Geometry: final body of the model. Coordinates: model frame, mm. Round coordinates to 2 decimals unless told otherwise and drop trailing zeros. Loops run counter-clockwise (first coordinate to the right, second up) from the corner with the lowest first, then second, coordinate; pieces in that order, holes last. Notation, with made-up numbers: (-39.75, 15.25) - (18.25, 15.25) arc R10 cw to (18.25, 32.25) - close; hole circle Ø7 at (11.25, 29.25). An arc over 180 degrees is marked (long way). Return JSON: item names as keys, results as strings. Group by question number.
1. Section D-D on x = 19.5. Return loops of the section in (y, z) (1 decimal), and give its area (3 significant figures).
2. Material intervals for probe 1 along Z at (x, y) = (36, 60.5); probe 2 along X at (y, z) = (137, 3.5), sorted ascending.
3. Section B-B on z = 17.75. Return loops of the section in (x, y) (1 decimal), and give its area (3 significant figures).
4. First-contact query: pin 1 Ø4 at (x, z) = (9, 21.5) entering from -Y. Flat tip, straight axial feed; report the tip coordinate or a pass-through.
5. Section A-A on x = 4. Return loops of the section in (y, z) (1 decimal), and give its area (3 significant figures).
6. Draft query along Z for faces 1 (the face through (25, 114, 25.4)), 2 (the face through (0.805, 215.193, 13.024)), 3 (the face through (50.017, 113.593, 13.024)), 4 (the face through (12.376, 11.993, 24.595)). Return one class per face: +Z half, -Z half, draft (parallel to the pull), parting line (faces both ways), or undercut.
7. Section C-C on y = 117.5. Return loops of the section in (x, z).
from build123d import *

# Parameters (mm, degrees)
SKETCH1_W           = 50.8
SKETCH1_H           = 225.425
SKETCH1_R           = 15.875
SKETCH1_R_2         = 2.4892
BOSS_EXTRUDE1_DEPTH = 25.4
SKETCH2_R           = 2.4892
CUT_EXTRUDE1_DEPTH  = 233.469848851
SKETCH3_W           = 47.625
SKETCH3_H           = 22.225
CUT_EXTRUDE2_DEPTH  = 233.469848884


with BuildPart() as part:
    # Sketch1 → Boss-Extrude1 (new body)
    with BuildSketch(Plane.XY):
        with Locations((25.4, 112.7125)):
            Rectangle(SKETCH1_W, SKETCH1_H)
        with Locations((25.4, 196.85)):
            Circle(SKETCH1_R, mode=Mode.SUBTRACT)
        with Locations((25.4, 9.525)):
            Circle(SKETCH1_R_2, mode=Mode.SUBTRACT)
        with Locations((38.1, 9.525)):
            Circle(SKETCH1_R_2, mode=Mode.SUBTRACT)
        with Locations((12.7, 9.525)):
            Circle(SKETCH1_R_2, mode=Mode.SUBTRACT)
        with Locations((12.7, 22.225)):
            Circle(SKETCH1_R_2, mode=Mode.SUBTRACT)
        with Locations((25.4, 22.225)):
            Circle(SKETCH1_R_2, mode=Mode.SUBTRACT)
        with Locations((38.1, 22.225)):
            Circle(SKETCH1_R_2, mode=Mode.SUBTRACT)
        with Locations((12.7, 34.925)):
            Circle(SKETCH1_R_2, mode=Mode.SUBTRACT)
        with Locations((25.4, 34.925)):
            Circle(SKETCH1_R_2, mode=Mode.SUBTRACT)
        with Locations((38.1, 34.925)):
            Circle(SKETCH1_R_2, mode=Mode.SUBTRACT)
        with Locations((12.7, 85.725)):
            Circle(SKETCH1_R_2, mode=Mode.SUBTRACT)
        with Locations((25.4, 85.725)):
            Circle(SKETCH1_R_2, mode=Mode.SUBTRACT)
        with Locations((38.1, 85.725)):
            Circle(SKETCH1_R_2, mode=Mode.SUBTRACT)
        with Locations((12.7, 98.425)):
            Circle(SKETCH1_R_2, mode=Mode.SUBTRACT)
        with Locations((25.4, 98.425)):
            Circle(SKETCH1_R_2, mode=Mode.SUBTRACT)
        with Locations((38.1, 98.425)):
            Circle(SKETCH1_R_2, mode=Mode.SUBTRACT)
        with Locations((12.7, 149.225)):
            Circle(SKETCH1_R_2, mode=Mode.SUBTRACT)
        with Locations((25.4, 149.225)):
            Circle(SKETCH1_R_2, mode=Mode.SUBTRACT)
        with Locations((38.1, 149.225)):
            Circle(SKETCH1_R_2, mode=Mode.SUBTRACT)
        with Locations((12.7, 161.925)):
            Circle(SKETCH1_R_2, mode=Mode.SUBTRACT)
        with Locations((25.4, 161.925)):
            Circle(SKETCH1_R_2, mode=Mode.SUBTRACT)
        with Locations((38.1, 161.925)):
            Circle(SKETCH1_R_2, mode=Mode.SUBTRACT)
    extrude(amount=BOSS_EXTRUDE1_DEPTH)

    # Sketch2 → Cut-Extrude1 (cut, through all)
    with BuildSketch(Plane(origin=(50.8, 0, 0), x_dir=(0, 0, -1), z_dir=(1, 0, 0))):
        with Locations((-12.7, 9.525)):
            Circle(SKETCH2_R)
        with Locations((-12.7, 22.225)):
            Circle(SKETCH2_R)
        with Locations((-12.7, 34.925)):
            Circle(SKETCH2_R)
        with Locations((-12.7, 47.625)):
            Circle(SKETCH2_R)
        with Locations((-12.7, 60.325)):
            Circle(SKETCH2_R)
        with Locations((-12.7, 73.025)):
            Circle(SKETCH2_R)
        with Locations((-12.7, 85.725)):
            Circle(SKETCH2_R)
        with Locations((-12.7, 98.425)):
            Circle(SKETCH2_R)
        with Locations((-12.7, 111.125)):
            Circle(SKETCH2_R)
        with Locations((-12.7, 123.825)):
            Circle(SKETCH2_R)
        with Locations((-12.7, 136.525)):
            Circle(SKETCH2_R)
        with Locations((-12.7, 149.225)):
            Circle(SKETCH2_R)
        with Locations((-12.7, 161.925)):
            Circle(SKETCH2_R)
        with Locations((-12.7, 174.625)):
            Circle(SKETCH2_R)
        with Locations((-12.7, 187.325)):
            Circle(SKETCH2_R)
        with Locations((-12.7, 200.025)):
            Circle(SKETCH2_R)
        with Locations((-12.7, 212.725)):
            Circle(SKETCH2_R)
    extrude(amount=-CUT_EXTRUDE1_DEPTH, mode=Mode.SUBTRACT)

    # Sketch3 → Cut-Extrude2 (cut, through all)
    with BuildSketch(Plane(origin=(0, 225.425, 0), x_dir=(1, 0, 0), z_dir=(0, 1, 0))):
        with Locations((25.4, -12.7)):
            Rectangle(SKETCH3_W, SKETCH3_H)
    extrude(amount=-CUT_EXTRUDE2_DEPTH, mode=Mode.SUBTRACT)


solid = part.part
Taken from the geometry:
{
 "1": {"outline": "(0, 0) - (182.1, 0) - (182.1, 1.6) - (0, 1.6) - close; (0, 23.8) - (182.1, 23.8) - (182.1, 25.4) - (0, 25.4) - close; (211.6, 0) - (225.4, 0) - (225.4, 1.6) - (211.6, 1.6) - close; (211.6, 23.8) - (225.4, 23.8) - (225.4, 25.4) - (211.6, 25.4) - close", "area": "622 mm2"},
 "2": {"probe 1": "0 to 1.59, 23.81 to 25.4", "probe 2": "0 to 1.59, 49.21 to 50.8"},
 "3": {"outline": "(0, 0) - (1.6, 0) - (1.6, 225.4) - (0, 225.4) - close; (49.2, 0) - (50.8, 0) - (50.8, 225.4) - (49.2, 225.4) - close", "area": "716 mm2"},
 "4": {"pin 1": "through"},
 "5": {"outline": "(0, 0) - (225.4, 0) - (225.4, 1.6) - (0, 1.6) - close; (0, 23.8) - (225.4, 23.8) - (225.4, 25.4) - (0, 25.4) - close", "area": "716 mm2"},
 "6": {"face 1": "+Z half", "face 2": "undercut", "face 3": "undercut", "face 4": "draft"},
 "7": {"outline": "(0, 0) - (50.8, 0) - (50.8, 25.4) - (0, 25.4) - close; hole (1.59, 1.59) - (49.21, 1.59) - (49.21, 23.81) - (1.59, 23.81) - close"}
}
